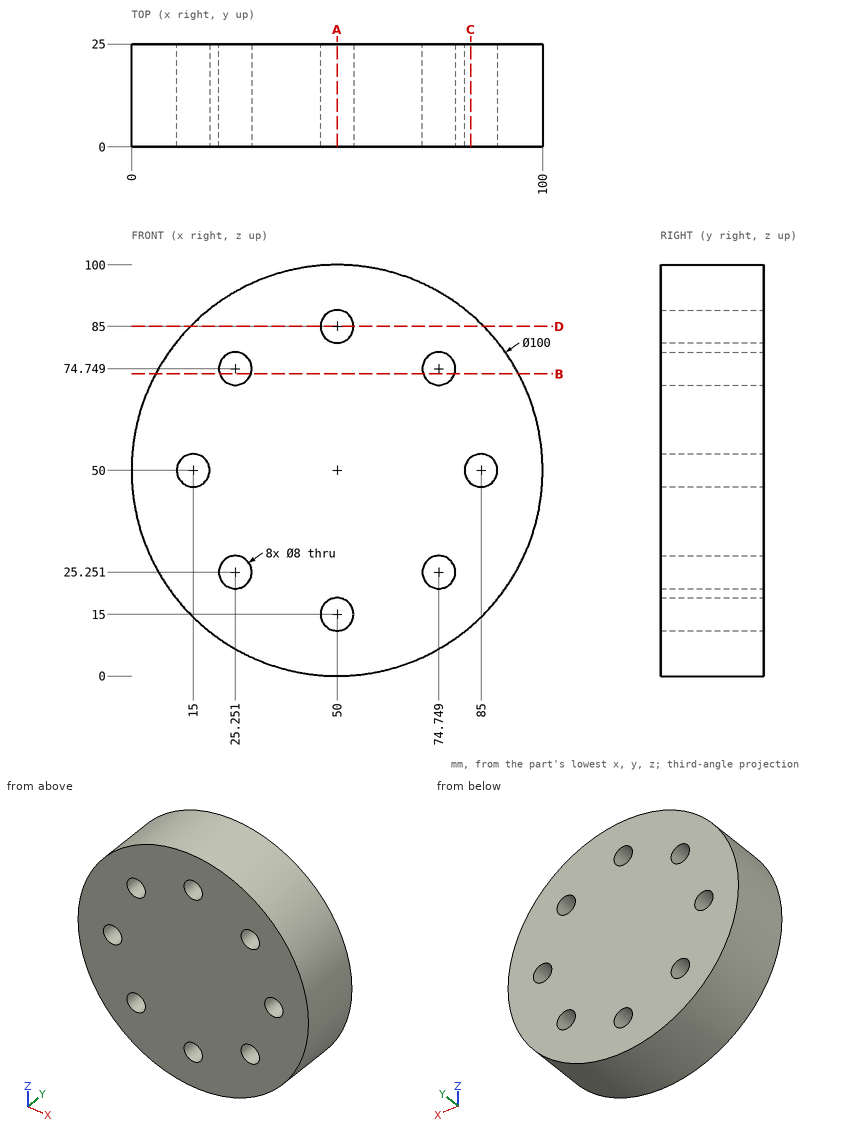
Input: dimensioned drawing with shaded views. Units: mm. Origin: part minimum x, y, z. Coordinates: 2 decimals unless noted, no trailing zeros. Order: outer loops, then holes, each group sorted by start corner. A loop starts at its lowest first (then second) coordinate and runs counter-clockwise, first axis right, second up. Notation, with made-up numbers: (15.25, -6.5) -> (35.25, -6.5) arc R31 ccw to (35.25, 29.5) -> close; hole circle Ø1 at (45.5, -32). An arc over 180 degrees is marked (long way). Answer in a Markdown table with one row per item.
Item 1: Section B-B on z = 73.5. Output: boundary loops of the cut face in (x, y), plus the area to 3 significant figures.
Return value:
| item | result |
|---|---|
| outline | (5.87, 0) -> (21.45, 0) -> (21.45, 25) -> (5.87, 25) -> close; (29.05, 0) -> (70.95, 0) -> (70.95, 25) -> (29.05, 25) -> close; (78.55, 0) -> (94.13, 0) -> (94.13, 25) -> (78.55, 25) -> close |
| area | 1,830 mm² |
Item 2: Ray query, L1, parallel to Z at x = 50, y = 11.75; L2, parallel to X at y = 15.5, z = 25.5 (1 decimal); L3, parallel to X at y = 21.25, z = 48 (1 decimal). Return the intervals inside material, ascending.
Return value:
| item | result |
|---|---|
| L1 | z = 0 to 11, 19 to 81, 89 to 100 |
| L2 | x = 6.4 to 21.3, 29.2 to 70.8, 78.7 to 93.6 |
| L3 | x = 0 to 11.5, 18.5 to 81.5, 88.5 to 100 |
Item 3: Section D-D on z = 85. Output: boundary loops of the cut face in (x, y), plus the area to 3 significant figures.
Return value:
| item | result |
|---|---|
| outline | (14.29, 0) -> (46, 0) -> (46, 25) -> (14.29, 25) -> close; (54, 0) -> (85.71, 0) -> (85.71, 25) -> (54, 25) -> close |
| area | 1,590 mm² |
Item 4: Contact query for flat-ended pins moving along their axis: P1, Ø5, axis at y = 3, z = 55.5, coming from the +X side; P2, Ø8, axis at y = 20.5, z = 44, coming from the +X side; P3, Ø4, axis at y = 6, z = 76.5, coming from the -X side. Output: stop coordinate, or through.
Return value:
| item | result |
|---|---|
| P1 | stops at x = 99.91 |
| P2 | stops at x = 99.96 |
| P3 | stops at x = 6.41 |
Item 5: Section C-C on x = 82.5. Output: boundary loops of the cut face in (y, z).
Return value:
| item | result |
|---|---|
| outline | (0, 12) -> (25, 12) -> (25, 46.88) -> (0, 46.88) -> close; (0, 53.12) -> (25, 53.12) -> (25, 88) -> (0, 88) -> close |
Item 6: Section A-A on x = 50. Output: boundary loops of the cut face in (y, z).
Return value:
| item | result |
|---|---|
| outline | (0, 0) -> (25, 0) -> (25, 11) -> (0, 11) -> close; (0, 19) -> (25, 19) -> (25, 81) -> (0, 81) -> close; (0, 89) -> (25, 89) -> (25, 100) -> (0, 100) -> close |
